from build123d import *

# Parameters (mm, degrees)
SKETCH1_R      = 1
EXTRUDE1_DEPTH = 5
FILLET2_R      = 1.8
FILLET3_R      = 1.2
SKETCH3_R      = 1.5
EXTRUDE2_DEPTH = 17


with BuildPart() as part:
    # Sketch1 → Extrude1 (new body)
    with BuildSketch(Plane.XY):
        Polygon((7.038618211, 6.213258786), (7.038618211, 16.213258786), (19.038618211, 36.213258786), (31.038618211, 36.213258786), (31.038618211, 33.213258786), (23.538618211, 33.213258786), (23.538618211, 27.213258786), (31.038618211, 27.213258786), (31.038618211, 24.213258786), (23.538618211, 24.213258786), (23.538618211, 13.213258786), (19.038618211, 6.213258786), align=None)
        with Locations((9.038618211, 9.738237996)):
            Circle(SKETCH1_R, mode=Mode.SUBTRACT)
        with Locations((19.038618211, 9.738237996)):
            Circle(SKETCH1_R, mode=Mode.SUBTRACT)
    extrude(amount=EXTRUDE1_DEPTH)

    # Fillet2
    fillet2_edges = [part.edges().sort_by_distance(p)[0] for p in [
        (7.038618211, 6.213258786, 2.5),
        (7.038618211, 16.213258786, 2.5),
        (19.038618211, 36.213258786, 2.5),
        (23.538618211, 13.213258786, 2.5),
        (19.038618211, 6.213258786, 2.5),
    ]]
    fillet(fillet2_edges, radius=FILLET2_R)

    # Fillet3
    fillet3_edges = [part.edges().sort_by_distance(p)[0] for p in [
        (23.538618211, 24.213258786, 2.5),
    ]]
    fillet(fillet3_edges, radius=FILLET3_R)

    # Sketch3 → Extrude2 (cut)
    with BuildSketch(Plane(origin=(0, 36.213258786, 0), x_dir=(1, 0, 0), z_dir=(0, 1, 0))):
        with Locations((29.038618211, -2.5)):
            Circle(SKETCH3_R)
    extrude(amount=-EXTRUDE2_DEPTH, mode=Mode.SUBTRACT)


solid = part.part
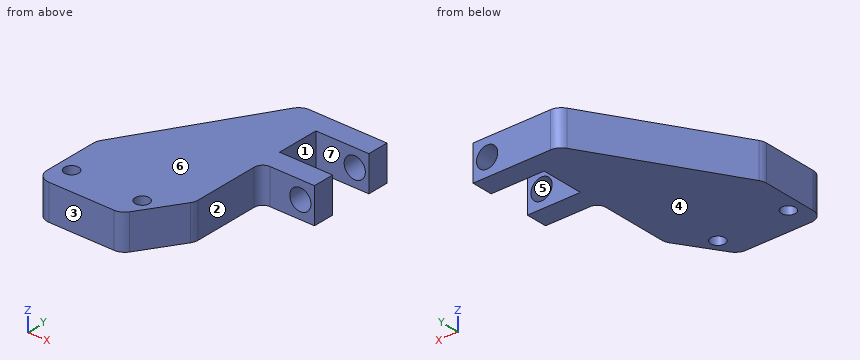
Input: part model. Units: mm. Frame: model coordinates. Face numbers are marked on the shaded views. A direction names the side the tool comes from. Coordinates: 2 decimals unless noted, no trailing zeros. Write each loop counter-clockwise with the first axis right and the second up, starting at its lowest first coordinate (ties: lowest second). Pieces come first, ordered by that corner, then holes. Notation, with made-up numbers: M -33,-24 L -5,-24 A18 cw -5,-2 Z; hole C -33,14 d4. An arc over 180 degrees is marked long. Answer as a JSON object with one key per item and string values. Group by question number.
(1) Section C-C on x = 21.5. Output: boundary loops of the cut face in (y, z).
(2) Section A-A on z = 2.5. Output: boundary loops of the cut face in (x, y).
(3) Contact query for flat-ended pins moving along their axis: P1, Ø10, axis at x = 28.5, y = 11, coming from the +Z side; P2, Ø1, axis at x = 20.5, z = 1.5, coming from the -Y side; P3, Ø2.5, axis at x = 26.5, z = 2.5, coming from the -Y side. Output: stop coordinate, or through.
(4) Set-up query: the marked faces 1, 2 and 3. Return all of +Z, -Z, +X, -X, +Y, -Y with unobstructed straight access to the full face (end or side cutting, diameter ignored); none if empty.
(5) Ray query, line 1 along Y through (x, z) = (25.5, 0.9); line 2 along X through (y, z) = (26.3, 2.5); line 3 along X through (y, z) = (34.1, 2.5). Return the intervals inside material, ascending. Write a range as [from, to].
(6) Section B-B on y = 14.5. Output: boundary loops of the cut face in (x, z), plus the area to 3 significant figures.
(7) Mould query, pull axis Z, two halves, no side actions, for the marked faces 4, 5, 6 and 7. Classes: pulls with the +Z half, pulls with the -Z half, needs draft (parallel to the pull), parting line crosses it, or undercut.
Result set:
{
 "1": {"outline": "M 10.04,0 L 36.21,0 L 36.21,5 L 10.04,5 Z"},
 "2": {"outline": "M 7.04,8.01 A1.8 ccw 8.84,6.21 L 18.06,6.21 A1.8 ccw 19.57,7.04 L 23.25,12.77 A1.8 ccw 23.54,13.74 L 23.54,23.01 A1.2 cw 24.74,24.21 L 27.54,24.21 L 27.54,27.21 L 23.54,27.21 L 23.54,33.21 L 27.54,33.21 L 27.54,36.21 L 20.06,36.21 A1.8 ccw 18.51,35.34 L 7.3,16.64 A1.8 ccw 7.04,15.71 Z; M 30.54,24.21 L 31.04,24.21 L 31.04,27.21 L 30.54,27.21 Z; M 30.54,33.21 L 31.04,33.21 L 31.04,36.21 L 30.54,36.21 Z; hole C 9.04,9.74 d2; hole C 19.04,9.74 d2"},
 "3": {"P1": "passes through", "P2": "stops at y = 7.71", "P3": "stops at y = 24.21"},
 "4": {"face 1": "+Z, -Z, +X", "face 2": "+Z, -Z, +X, -Y", "face 3": "+Z, -Z, +X, -X, -Y"},
 "5": {"line 1": "y = [24.21, 27.21], [33.21, 36.21]", "line 2": "x = [13.09, 27.54], [30.54, 31.04]", "line 3": "x = [17.77, 27.54], [30.54, 31.04]"},
 "6": {"outline": "M 7.04,0 L 23.54,0 L 23.54,5 L 7.04,5 Z", "area": "82.5 mm2"},
 "7": {"face 4": "pulls with the -Z half", "face 5": "undercut", "face 6": "pulls with the +Z half", "face 7": "needs draft"}
}
